The listing builds one solid part. Answer for the finished solid, in the listing's coordinates (mm). Face numbers are marked on the shaded views. A direction names the side the tool comes from. Coordinates: 2 decimals unless noted, no trailing zeros. Order: outer loops, then holes, each group sorted by start corner. A loop starts at its lowest first (then second) coordinate and runs counter-clockwise, first axis right, second up. Notation, with made-up numbers: (-9.75, 24.25) -> (34.25, 24.25) arc R30 ccw to (34.25, 57.25) -> close; hole circle Ø7 at (58, 26.25). An arc over 180 degrees is marked (long way). Write item = value, one per line. Start each with the question number.
Autodesk Inventor part; units mm, degrees
ref_plane "Work Plane1" through (33.575, 0, 0) normal (0, 0, -1) x (1, 0, 0)
ref_plane "YZ Plane" through (0, 0, 0) normal (1, 0, 0) x (0, 1, 0)
ref_plane "XZ Plane" through (0, 0, 0) normal (0, 1, 0) x (-1, 0, 0)
sketch "Sketch1" plane through (0, 0, 0) normal (0, 0, 1) x (1, 0, 0)
  line L0 (0, 0) -> (25.4, 0)
  line L1 (25.4, 0) -> (25.4, 3.175)
  line L2 (25.4, 3.175) -> (6.731, 3.175)
  line L3 (6.731, 3.175) -> (5.461, 3.175)
  line L4 (5.461, 3.175) -> (3.556, 3.175)
  line L5 (3.556, 3.175) -> (0.6048, 5.7404)
  line L6 (0.6048, 5.7404) -> (0, 5.7404)
  line L7 (0, 5.7404) -> (0, 0)
  line L8 (6.731, 3.175) -> (3.556, 3.175) construction
  line L9 (-5.08, 0) -> (30.48, 0)
  line L10 (0, 6.8885) -> (0, -1.1481)
  dimension "d0" = 25.4
  dimension "d1" = 41
  dimension "d2" = 1.27
  dimension "d3" = 18.669
  dimension "d4" = 3.556
  dimension "d5" = 6.35
  dimension "d6" = 6.35
  dimension "d7" = 11.4808
revolve "Body" add sketch "Sketch1" angle 360 about axis through (0, 0, 0) along (1, 0, 0)
sketch "Sketch2" plane through (0, 0, 0) normal (-1, 0, 0) x (0, 0, 1)
  line L0 (5.7404, -0.9525) -> (-5.7404, -0.9525)
  line L1 (-5.7404, -0.9525) -> (-5.7404, 0.9525)
  line L2 (-5.7404, 0.9525) -> (5.7404, 0.9525)
  line L3 (5.7404, 0.9525) -> (5.7404, -0.9525)
  line L4 (0, 0.9525) -> (0, -0.9525) construction
  line L5 (-5.7404, 0) -> (5.7404, 0) construction
  line L6 (0, 5.7404) -> (0, 0)
  dimension "d15" = 1.905
  dimension "d16" = 11.4808
extrude "Slot" cut sketch "Sketch2" against normal blind 1.7272
thread "Thread"
chamfer "Chamfer1" distance 0.7556 distance2 0.635 1 edges at (25.4, -3.175, 0) measured on face at (25.4, 0.7614, 0.4485)
fillet "Radius" radius 2.54 1 edges at (3.556, -3.175, 0)
ref_plane "Work Plane1" through (33.575, 0, 0) normal (0, 0, -1) x (1, 0, 0)
equation "\"d0\" = NLG"
equation "\"d1\" = 0.5 * SEWI"
equation "\"d2\" = GAL"
equation "\"d3\" = GEL"
equation "\"d4\" = KOH"
equation "\"d5\" = BDM"
equation "\"d6\" = GD"
equation "\"d7\" = KOD"
equation "\"d15\" = SBR"
equation "\"d16\" = KOD"
equation "\"d8\" = STI"
equation "\"d41\" = RR"
equation "\"d10\" = GEL"
equation "\"d12\" = -0.5 * SPD + 0.5 * GD"
equation "\"d13\" = 0.5 * GAL"
equation "\"NLG\" = 25.4"
equation "\"GAL\" = 1.27"
equation "\"GEL\" = 18.669"
equation "\"KOH\" = 3.556"
equation "\"KOD\" = 11.4808"
equation "\"SEWI\" = 82deg"
equation "\"BDM\" = NND"
equation "\"GD\" = NND"
equation "\"SBR\" = 1.905"
equation "\"STI\" = 1.7272"
equation "\"SPD\" = 4.8387"
equation "\"RR\" = 2.54"
equation "\"GUL\" = 0.75565"
equation "\"TOA\" = 30deg"
equation "\"THREADDIA\" = 6.35"
equation "\"HHPTC\" = 1.27"
equation "\"NND\" = 6.35"
equation "\"GD1\" = SPD"
properties part number "ANSI B18.6.2 - 1/4-20 UNC x 1, SFCHCSI" material "Steel, Mild"
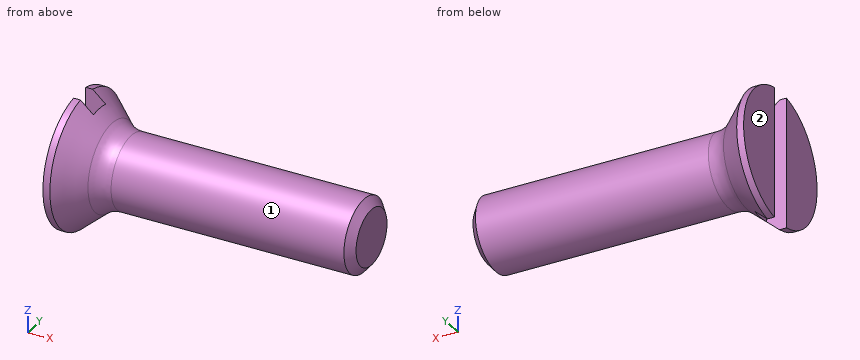
Item 1: Consider probe 1 along Z at (x, y) = (24.25, 0) (3 decimals); probe 2 along X at (y, z) = (-0.75, 2.25); probe 3 along X at (y, z) = (-3.25, 1.75). Determine where each line is inside the solid, lowest interval first.
Item 2: Section A-A, the plane x = 6 is taken. Give the vertices of the cut face in (y, z) (3 decimals).
Item 3: Which of the six approach directions +Z, -Z, +X, -X, +Y, -Y give full straight-line access (tool end or side, diameter ignored) to the marked faces 1 and 2?
Item 4: Each of these flat-tipped pins is pushed along its axis until it touches: pin 1 (1 mm diameter, centred on y = 4, z = 2.5, fed in from -X); pin 2 (0.5 mm diameter, centred on x = 1, z = 1.5, fed in from -Y); pin 3 (1.5 mm diameter, centred on x = 4, y = -2, fed in from +Z); pin 4 (1.4 mm diameter, centred on x = 1, z = 1, fed in from +Y). Where does it stop, or does it pass through?
A:
q1.probe_1 = -3.175 to 3.175
q1.probe_2 = 1.73 to 25.4
q1.probe_3 = 0 to 2.97
q2.outline = circle Ø6.35 at (0, 0)
q3.face_1 = +X
q3.face_2 = +Z, -Z, -X, +Y, -Y
q4.pin_1 = 0
q4.pin_2 = -5.42
q4.pin_3 = 3.06
q4.pin_4 = 5.72
